from build123d import *

# Parameters (mm, degrees)
F0_R     = 1
F1_DEPTH = 4
F3_COUNT = 12


with BuildPart() as f1:
    # F0 (on Top) → F1 (new body)
    with BuildSketch(Plane.XY):
        with BuildLine():
            Line((8.6503619001, 0.5578879787), (8.2103695235, 2.1999618834))
            Line((8.2103695235, 2.1999618834), (6.761480784, 1.8117333157))
            ThreePointArc((6.761480784, 1.8117333157), (7, 0), (6.761480784, -1.8117333157))
            Line((6.761480784, -1.8117333157), (8.2103695235, -2.1999618834))
            Line((8.2103695235, -2.1999618834), (8.6503619001, -0.5578879787))
            Line((8.6503619001, -0.5578879787), (12.5140652053, -1.5931641591))
            ThreePointArc((12.5140652053, -1.5931641591), (13.6406023857, -1.1265371804), (14.1072293644, 0))
            ThreePointArc((14.1072293644, 0), (13.6406023857, 1.1265371804), (12.5140652053, 1.5931641591))
            Line((12.5140652053, 1.5931641591), (8.6503619001, 0.5578879787))
        make_face()
        with Locations((12.5140652053, 0)):
            Circle(F0_R, mode=Mode.SUBTRACT)
    extrude(amount=F1_DEPTH)

    # F3: F1 ×12 about axis
    f3_axis = Axis((0, 0, -5.4754605517), (0, 0, -1))


with BuildPart() as f1_1:
    add(f1.part)
    for i in range(1, F3_COUNT):
        add(f1.part.rotate(f3_axis, i * 360 / F3_COUNT))


solid = f1_1.part
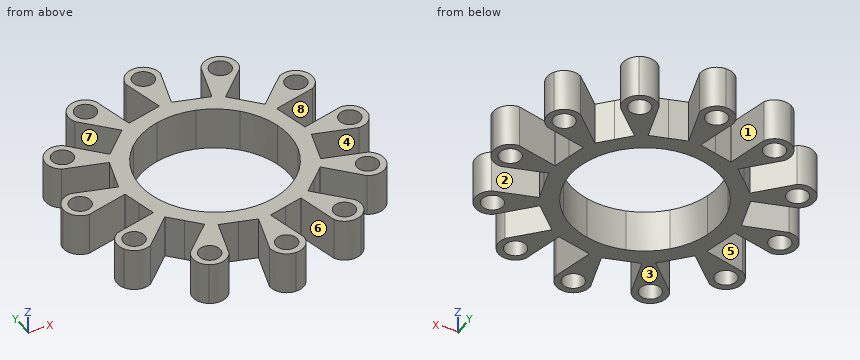
Input: part model. Units: mm. Frame: model coordinates. Face numbers are marked on the shaded views. A direction names the side the tool comes from. Coordinates: 2 decimals unless noted, no trailing zeros.
Q1. Material intervals for line 1 (Y direction, x = -11.25, z = 1.15); line 2 (X direction, y = -10.75, z = 3.5); line 3 (Y direction, x = 11, z = 0.6), sorted ascending.
Q2. Cut plane A-A (z = 3.05). Give the number of separate pieces and of enclosed holes in the cut face, then the cut area to 3 significant figures.
Q3. Contact query for flat-ended pins moving along their axis: pin 1 (3 mm diameter, centred on x = -6.26, y = 10.84, fed in from -Z); pin 2 (1 mm diameter, centred on y = -6.5, z = 3, fed in from -X). Output: stop coordinate, or through.
Q4. Draft query along Y for the marked faces 1, 2, 3 and 4. Return one class per face: +Y half, -Y half, draft (parallel to the pull), parting line (faces both ways), or undercut.
Q5. Set-up query: the marked faces 5, 6, 7 and 8. Return all of +Z, -Z, +X, -X, +Y, -Y with unobstructed straight access to the full face (end or side cutting, diameter ignored); none if empty.
Working result:
1. line 1: y = -7.8 to -7.17, -5.35 to -4.77, -1.25 to 1.25, 4.77 to 5.35, 7.17 to 7.8
1. line 2: x = -7.85 to -7.25, -5.26 to -4.64, -1.12 to 1.12, 4.64 to 5.26, 7.25 to 7.85
1. line 3: y = -7.84 to -7.24, -5.27 to -4.71, -1.19 to 1.19, 4.71 to 5.27, 7.24 to 7.84
2. separate pieces: 1
2. enclosed holes: 13
2. area: 187 mm2
3. pin 1: stops at z = 0
3. pin 2: stops at x = -12.43
4. face 1: +Y half
4. face 2: undercut
4. face 3: draft
4. face 4: undercut
5. face 5: +Z, -Z, -X
5. face 6: +Z, -Z, -Y
5. face 7: +Z, -Z
5. face 8: +Z, -Z, +X
